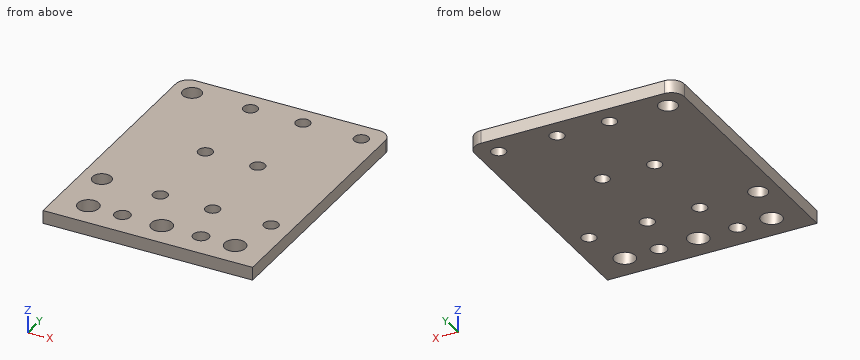
from build123d import *

# Parameters (mm, degrees)
F0_R     = 4
F0_R_2   = 3
F0_R_3   = 3.5685
F0_R_4   = 2.75
F1_DEPTH = 5


with BuildPart() as f1:
    # F0 (on Top) → F1 (new body)
    with BuildSketch(Plane.XY):
        with BuildLine():
            Line((40, 0), (5, 0))
            ThreePointArc((5, 0), (1.464466, -1.464466), (0, -5))
            Line((0, -5), (0, -100))
            Line((0, -100), (80, -100))
            Line((80, -100), (80, -5))
            ThreePointArc((80, -5), (78.535534, -1.464466), (75, 0))
            Line((75, 0), (40, 0))
        make_face()
        with Locations((12, -90)):
            Circle(F0_R, mode=Mode.SUBTRACT)
        with Locations((25, -90)):
            Circle(F0_R_2, mode=Mode.SUBTRACT)
        with Locations((7.7, -72.3)):
            Circle(F0_R_3, mode=Mode.SUBTRACT)
        with Locations((30, -72.3)):
            Circle(F0_R_4, mode=Mode.SUBTRACT)
        with Locations((40, -90)):
            Circle(F0_R, mode=Mode.SUBTRACT)
        with Locations((55, -90)):
            Circle(F0_R_2, mode=Mode.SUBTRACT)
        with Locations((68, -90)):
            Circle(F0_R, mode=Mode.SUBTRACT)
        with Locations((50, -72.3)):
            Circle(F0_R_4, mode=Mode.SUBTRACT)
        with Locations((72.3, -72.3)):
            Circle(F0_R_4, mode=Mode.SUBTRACT)
        with Locations((30, -40)):
            Circle(F0_R_4, mode=Mode.SUBTRACT)
        with Locations((7.7, -7.7)):
            Circle(F0_R_3, mode=Mode.SUBTRACT)
        with Locations((30, -7.7)):
            Circle(F0_R_4, mode=Mode.SUBTRACT)
        with Locations((50, -40)):
            Circle(F0_R_4, mode=Mode.SUBTRACT)
        with Locations((50, -7.7)):
            Circle(F0_R_4, mode=Mode.SUBTRACT)
        with Locations((72.3, -7.7)):
            Circle(F0_R_4, mode=Mode.SUBTRACT)
    extrude(amount=F1_DEPTH)


solid = f1.part
Here's how the part is built. I have some questions about the finished solid (model axes, mm). Round coordinates to 2 decimals unless told otherwise and drop trailing zeros. Write each loop counter-clockwise with the first axis right and the second up, starting at its lowest first coordinate (ties: lowest second). Pieces come first, ordered by that corner, then holes. Notation, with made-up numbers: (34.5, 88) -> (40.5, 88) arc R20 ccw to (40.5, 108) -> close; hole circle Ø7 at (77, 69). An arc over 180 degrees is marked (long way). One line per item, written item: value.
1) If I drill on line 1 (Y direction, x = 50, z = 3.8); line 2 (Y direction, x = 31, z = 3.8); line 3 (Y direction, x = 25, z = 3.65), over which ranges is the centre line in solid material (lowest first)? Write a range as [from, to].
Filled sheet:
line 1: y = [-100, -75.05], [-69.55, -42.75], [-37.25, -10.45], [-4.95, 0]
line 2: y = [-100, -74.86], [-69.74, -42.56], [-37.44, -10.26], [-5.14, 0]
line 3: y = [-100, -93], [-87, 0]
2) I'm going to push a flat-ended pin straight in: pin 1 Ø9 at (x, y) = (12, -90) entering from +Z. Where does the tip first touch, or does it pass through?
Filled sheet:
pin 1: stops at z = 5
3) Suppose I cut it at D-D on x = 40. List the corners of the cut face in (y, z) for me, plus the area to 3 significant figures.
Filled sheet:
outline: (-100, 0) -> (-94, 0) -> (-94, 5) -> (-100, 5) -> close; (-86, 0) -> (0, 0) -> (0, 5) -> (-86, 5) -> close
area: 460 mm2
4) Suppose I cut it at A-A on x = 30. List the corners of the cut face in (y, z) for me.
Filled sheet:
outline: (-100, 0) -> (-75.05, 0) -> (-75.05, 5) -> (-100, 5) -> close; (-69.55, 0) -> (-42.75, 0) -> (-42.75, 5) -> (-69.55, 5) -> close; (-37.25, 0) -> (-10.45, 0) -> (-10.45, 5) -> (-37.25, 5) -> close; (-4.95, 0) -> (0, 0) -> (0, 5) -> (-4.95, 5) -> close
5) Suppose I cut it at C-C on z = 1.85. Give the number of separate pieces and of enclosed holes in the cut face, plus the area to 3 significant figures.
Filled sheet:
separate pieces: 1
enclosed holes: 15
area: 7,510 mm2
6) Suppose I cut it at B-B on y = -40. List the corners of the cut face in (x, z) for me, plus the area to 3 significant figures.
Filled sheet:
outline: (0, 0) -> (27.25, 0) -> (27.25, 5) -> (0, 5) -> close; (32.75, 0) -> (47.25, 0) -> (47.25, 5) -> (32.75, 5) -> close; (52.75, 0) -> (80, 0) -> (80, 5) -> (52.75, 5) -> close
area: 345 mm2
